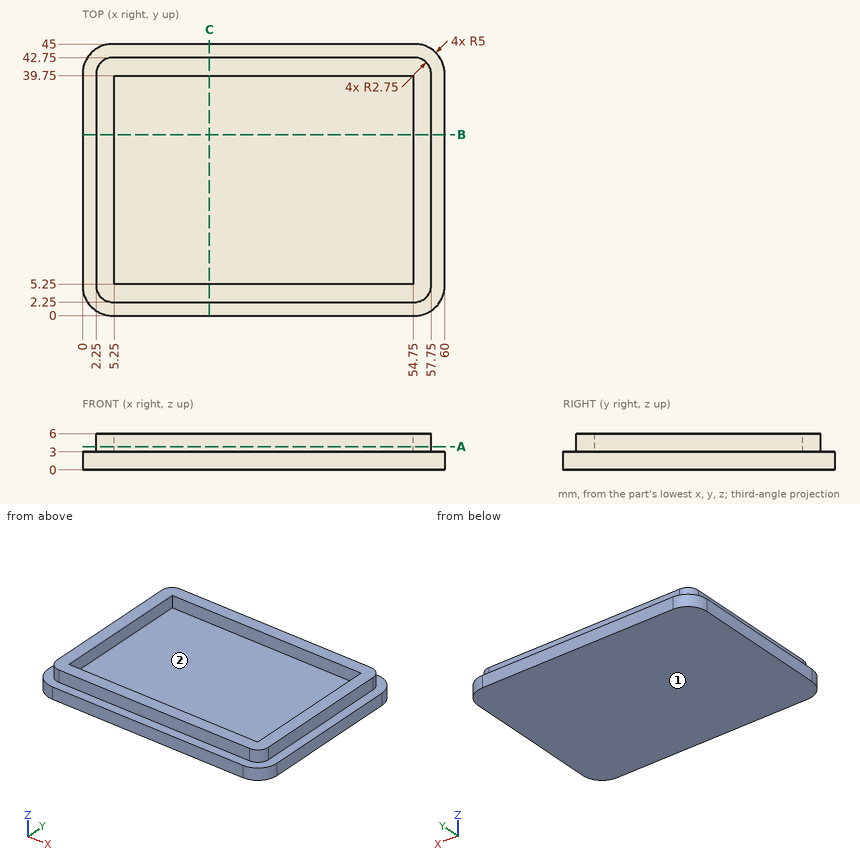
Job drawing, mm, ordinate dimensions from the low corner. One solid piece. Coordinates: 2 decimals unless noted, no trailing zeros. Write each loop counter-clockwise with the first axis right and the second up, starting at its lowest first coordinate (ties: lowest second). Pieces come first, ordered by that corner, then holes. Notation, with made-up numbers: (26, 87.25) - (63, 87.25) arc R26 ccw to (63, 118.25) - close; hole circle Ø10 at (-40, 54.5). An arc over 180 degrees is marked (long way). Use a Markdown table: item, result. Add a question column.
Item 1: Mould opens along X. For the marked faces 1 and 2 say: pulls with the +X half, pulls with the -X half, needs draft (parallel to the pull), parting line crosses it, or undercut.
Item 2: Flat gauge pins, fed straight in: pin 1 (0.9 mm diameter, centred on x = 28.5, z = 5, fed in from -Y); pin 2 (3.5 mm diameter, centred on y = 22, z = 4.5, fed in from -X); pin 3 (4 mm diameter, centred on x = 18.5, y = 13.5, fed in from +Z); pin 4 (0.9 mm diameter, centred on y = 25, z = 4.5, fed in from +X). Where does each tip first touch, or does it go through?
Item 3: Drill centre lines: L1, parallel to Y at x = 44, z = 3.2; L2, parallel to X at y = 22, z = 5.3; L3, parallel to Y at x = 55, z = 4.5. Where is each one in solid material? Low to high. Write a range as from..to.
Item 4: Band-saw the part on C-C, the plane x = 21. Give the cut face in (y, z), and give its area (3 significant figures).
Item 5: Band-saw the part on A-A, the plane z = 3.85. Give the cut face in (x, y).
Item 6: Band-saw the part on B-B, the plane y = 30. Give the cut face in (x, z), and give its area (3 significant figures).
Numbers:
| question | item | result |
|---|---|---|
| 1 | face 1 | needs draft |
| 1 | face 2 | undercut |
| 2 | pin 1 | y = 2.25 |
| 2 | pin 2 | x = 0 |
| 2 | pin 3 | z = 3 |
| 2 | pin 4 | x = 57.75 |
| 3 | L1 | 2.25..5.25, 39.75..42.75 |
| 3 | L2 | 2.25..5.25, 54.75..57.75 |
| 3 | L3 | 2.25..42.75 |
| 4 | outline | (0, 0) - (45, 0) - (45, 3) - (42.75, 3) - (42.75, 6) - (39.75, 6) - (39.75, 3) - (5.25, 3) - (5.25, 6) - (2.25, 6) - (2.25, 3) - (0, 3) - close |
| 4 | area | 153 mm2 |
| 5 | outline | (2.25, 5) arc R2.75 ccw to (5, 2.25) - (55, 2.25) arc R2.75 ccw to (57.75, 5) - (57.75, 40) arc R2.75 ccw to (55, 42.75) - (5, 42.75) arc R2.75 ccw to (2.25, 40) - close; hole (5.25, 5.25) - (54.75, 5.25) - (54.75, 39.75) - (5.25, 39.75) - close |
| 6 | outline | (0, 0) - (60, 0) - (60, 3) - (57.75, 3) - (57.75, 6) - (54.75, 6) - (54.75, 3) - (5.25, 3) - (5.25, 6) - (2.25, 6) - (2.25, 3) - (0, 3) - close |
| 6 | area | 198 mm2 |
